Check sheet for the drawn part. Datum: minimum x, y, z corner. Units: mm. A direction names the side the tool comes from. Give positions to 0.01 mm unless a question says otherwise; leave off trailing zeros. Order: outer loops, then holes, each group sorted by start corner. A loop starts at its lowest first (then second) coordinate and runs counter-clockwise, first axis right, second up. Notation, with made-up numbers: (16, 79) -> (60, 79) arc R16 cw to (60, 102) -> close; hole circle Ø6 at (37, 65.25). An arc over 180 degrees is marked (long way). Return JSON: item names as keys, results as strings. Group by question number.
(1) Cross-section at B-B on y = 30. Enter the section's corners in (x, z).
(2) Cross-section at D-D on x = 17.5. Enter the section's corners in (y, z).
(3) Tool access check on the marked faces 4 and 5. Record the directions out of +Z, -Z, +X, -X, +Y, -Y that give a thin tool (end or side, any length) a straight path to the whole face; none if there is none.
(4) Depth check by flat-ended pin: pin 1 Ø3 at (x, z) = (46, 5) entering from +Y; pin 2 Ø3 at (y, z) = (13, 3.5) entering from +X; pin 3 Ø1 at (y, z) = (52.5, 3) entering from -X. Enter the tip coordinate at first touch or a pass-through.
(5) Release check for a two-part mould opening along X. For the marked faces 1, 2 and 3 record: pulls with the +X half, pulls with the -X half, needs draft (parallel to the pull), parting line crosses it, or undercut.
(6) Cross-section at C-C on y = 50. Enter the section's corners in (x, z), then the cut area to 3 significant figures.
(7) Cross-section at A-A on x = 30. Enter the section's corners in (y, z).
(8) Thickness scan on line 1 along Y through (x, z) = (30, 7.8); line 2 along Y through (x, z) = (30, 4.5); line 3 along Z through (x, y) = (42.5, 19). Record the ranges inside material, lowest first.
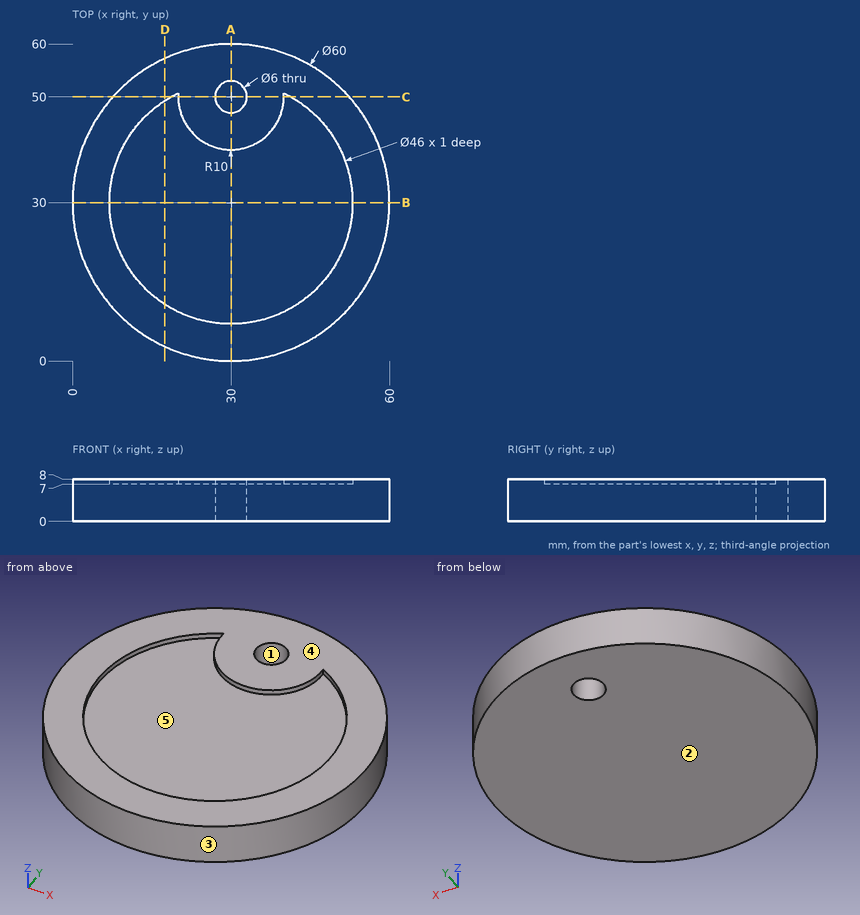
Verdict:
{
 "1": {"outline": "(0, 0) -> (60, 0) -> (60, 8) -> (53, 8) -> (53, 7) -> (7, 7) -> (7, 8) -> (0, 8) -> close"},
 "2": {"outline": "(2.73, 0) -> (57.27, 0) -> (57.27, 8) -> (49.31, 8) -> (49.31, 7) -> (10.69, 7) -> (10.69, 8) -> (2.73, 8) -> close"},
 "3": {"face 4": "+Z, +X, -X, +Y, -Y", "face 5": "+Z"},
 "4": {"pin 1": "y = 56.26", "pin 2": "x = 55.69", "pin 3": "x = 9.6"},
 "5": {"face 1": "undercut", "face 2": "needs draft", "face 3": "parting line crosses it"},
 "6": {"outline": "(7.64, 0) -> (27, 0) -> (27, 8) -> (20, 8) -> (20, 7) -> (18.64, 7) -> (18.64, 8) -> (7.64, 8) -> close; (33, 0) -> (52.36, 0) -> (52.36, 8) -> (41.36, 8) -> (41.36, 7) -> (40, 7) -> (40, 8) -> (33, 8) -> close", "area": "307 mm²"},
 "7": {"outline": "(0, 0) -> (47, 0) -> (47, 8) -> (40, 8) -> (40, 7) -> (7, 7) -> (7, 8) -> (0, 8) -> close; (53, 0) -> (60, 0) -> (60, 8) -> (53, 8) -> close"},
 "8": {"line 1": "0 to 7, 40 to 47, 53 to 60", "line 2": "0 to 47, 53 to 60", "line 3": "0 to 7"}
}
